from build123d import *

# Parameters (mm, degrees)
CROQUIS1_W              = 121.5
CROQUIS1_H              = 101
SALIENTE_EXTRUIR2_DEPTH = 4
SALIENTE_EXTRUIR3_DEPTH = 75
CROQUIS3_W              = 50
CROQUIS3_H              = 4
SALIENTE_EXTRUIR4_DEPTH = 75
CORTAR_EXTRUIR1_REACH   = 161.266
CROQUIS4_R              = 3.5
CROQUIS5_R              = 3.5
CORTAR_EXTRUIR2_DEPTH   = 4
CORTAR_EXTRUIR3_START   = -54.5
CORTAR_EXTRUIR3_DEPTH   = 109


with BuildPart() as part:
    # Croquis1 → Saliente-Extruir2 (new body)
    with BuildSketch(Plane(origin=(0, 0, 0), x_dir=(1, 0, 0), z_dir=(0, 1, 0))):
        Rectangle(CROQUIS1_W, CROQUIS1_H)
    extrude(amount=SALIENTE_EXTRUIR2_DEPTH)

    # Croquis2 → Saliente-Extruir3 (add)
    with BuildSketch(Plane(origin=(0, 0, 0), x_dir=(1, 0, 0), z_dir=(0, 1, 0))):
        Polygon((60.75, -50.5), (64.75, -50.5), (64.75, 54.5), (60.75, 54.5), (-64.75, 54.5), (-64.75, -50.5), (-60.75, -50.5), (-60.75, 50.5), (60.75, 50.5), align=None)
    extrude(amount=SALIENTE_EXTRUIR3_DEPTH)

    # Croquis3 → Saliente-Extruir4 (add)
    with BuildSketch(Plane(origin=(0, 0, 0), x_dir=(1, 0, 0), z_dir=(0, 1, 0))):
        with Locations((39.75, -52.5)):
            Rectangle(CROQUIS3_W, CROQUIS3_H)
    extrude(amount=SALIENTE_EXTRUIR4_DEPTH)

    # Cortar-Extruir1: up to this face of the body (flat: up to its plane)
    cortar_extruir1_end = Plane(part.part.faces().sort_by_distance((-64.75, 37.5, -2))[0])
    # Croquis4 → Cortar-Extruir1 (cut, up to the picked face)
    with BuildSketch(Plane(origin=(64.75, 0, 0), x_dir=(0, 0, -1), z_dir=(1, 0, 0)), mode=Mode.PRIVATE) as cortar_extruir1_sk1:
        with Locations((-35, 69.5)):
            Circle(CROQUIS4_R)
    cortar_extruir1_tool1 = split(extrude(cortar_extruir1_sk1.sketch, amount=-CORTAR_EXTRUIR1_REACH, mode=Mode.PRIVATE), bisect_by=cortar_extruir1_end, keep=Keep.BOTH, mode=Mode.PRIVATE)
    # Croquis4 → Cortar-Extruir1 (cut, up to the picked face)
    with BuildSketch(Plane(origin=(64.75, 0, 0), x_dir=(0, 0, -1), z_dir=(1, 0, 0)), mode=Mode.PRIVATE) as cortar_extruir1_sk2:
        with Locations((35, 9.5)):
            Circle(CROQUIS4_R)
    cortar_extruir1_tool2 = split(extrude(cortar_extruir1_sk2.sketch, amount=-CORTAR_EXTRUIR1_REACH, mode=Mode.PRIVATE), bisect_by=cortar_extruir1_end, keep=Keep.BOTH, mode=Mode.PRIVATE)
    # Croquis4 → Cortar-Extruir1 (cut, up to the picked face)
    with BuildSketch(Plane(origin=(64.75, 0, 0), x_dir=(0, 0, -1), z_dir=(1, 0, 0)), mode=Mode.PRIVATE) as cortar_extruir1_sk3:
        with Locations((-35, 9.5)):
            Circle(CROQUIS4_R)
    cortar_extruir1_tool3 = split(extrude(cortar_extruir1_sk3.sketch, amount=-CORTAR_EXTRUIR1_REACH, mode=Mode.PRIVATE), bisect_by=cortar_extruir1_end, keep=Keep.BOTH, mode=Mode.PRIVATE)
    # Croquis4 → Cortar-Extruir1 (cut, up to the picked face)
    with BuildSketch(Plane(origin=(64.75, 0, 0), x_dir=(0, 0, -1), z_dir=(1, 0, 0)), mode=Mode.PRIVATE) as cortar_extruir1_sk4:
        with Locations((35, 69.5)):
            Circle(CROQUIS4_R)
    cortar_extruir1_tool4 = split(extrude(cortar_extruir1_sk4.sketch, amount=-CORTAR_EXTRUIR1_REACH, mode=Mode.PRIVATE), bisect_by=cortar_extruir1_end, keep=Keep.BOTH, mode=Mode.PRIVATE)
    add(cortar_extruir1_tool1.solids().sort_by(Axis((64.75, 69.5, 35), (-1, 0, 0)))[0], mode=Mode.SUBTRACT)
    add(cortar_extruir1_tool2.solids().sort_by(Axis((64.75, 9.5, -35), (-1, 0, 0)))[0], mode=Mode.SUBTRACT)
    add(cortar_extruir1_tool3.solids().sort_by(Axis((64.75, 9.5, 35), (-1, 0, 0)))[0], mode=Mode.SUBTRACT)
    add(cortar_extruir1_tool4.solids().sort_by(Axis((64.75, 69.5, -35), (-1, 0, 0)))[0], mode=Mode.SUBTRACT)

    # Croquis5 → Cortar-Extruir2 (cut)
    with BuildSketch(Plane(origin=(0, 0, -54.5), x_dir=(-1, 0, 0), z_dir=(0, 0, -1))):
        with Locations((44.25, 69.5)):
            Circle(CROQUIS5_R)
        with Locations((44.25, 9.5)):
            Circle(CROQUIS5_R)
    extrude(amount=-CORTAR_EXTRUIR2_DEPTH, mode=Mode.SUBTRACT)

    # Croquis6 → Cortar-Extruir3 (cut)
    with BuildSketch(Plane.XY.offset(CORTAR_EXTRUIR3_START)):
        with BuildLine():
            Line((42.75, 69), (42.75, 75))
            Line((42.75, 75), (45.75, 75))
            Line((45.75, 75), (48.75, 75))
            Line((48.75, 75), (48.75, 69))
            ThreePointArc((48.75, 69), (45.75, 66), (42.75, 69))
        make_face()
        with BuildLine():
            ThreePointArc((48.75, 10), (47.871320344, 12.121320344), (45.75, 13))
            Line((45.75, 13), (45.75, 7))
            ThreePointArc((45.75, 7), (47.871320344, 7.878679656), (48.75, 10))
        make_face()
        with BuildLine():
            Line((45.75, 7), (45.75, 13))
            ThreePointArc((45.75, 13), (42.75, 10), (45.75, 7))
        make_face()
    extrude(amount=CORTAR_EXTRUIR3_DEPTH, mode=Mode.SUBTRACT)


solid = part.part
Design review of the part built by this model. Coordinates are the model's own, in mm. A direction names the side the tool comes from. Round coordinates to 2 decimals unless told otherwise and drop trailing zeros. Loops run counter-clockwise (first coordinate to the right, second up) from the corner with the lowest first, then second, coordinate; pieces in that order, holes last. Notation, with made-up numbers: M 82.25,50 L 105.25,50 A8 cw 105.25,54 Z; hole C 50.5,11.25 d10. An arc over 180 degrees is marked long. Answer as a JSON object with one key per item and string values.
Item 1: Machinability: for faces 4 (the flat face through (-37, 1, 50.5)), 5 (the flat face through (37, 39, 50.5)), 6 (the flat face through (39, 37, 54.5)), 7 (the flat face through (42.75, 72, -53)), 8 (the cylindrical face through (62.778, 69.654, 38.497)), which of the approach directions +Z, -Z, +X, -X, +Y, -Y give a long, thin tool a straight path to every point of the face, cutting with its end or side? Answer none if there is none.
Answer sheet:
{"face 4": "+Z, -X, +Y, -Y", "face 5": "+Y", "face 6": "+Z, +X, -X, +Y, -Y", "face 7": "+Z, -Z, +Y", "face 8": "+X, -X"}
Item 2: We need section D-D on z = -21. Give the boundary of the cut face in (x, y), and give its area (3 significant figures).
Answer sheet:
{"outline": "M -64.75,0 L 64.75,0 L 64.75,75 L 60.75,75 L 60.75,4 L -60.75,4 L -60.75,75 L -64.75,75 Z", "area": "1,090 mm^2"}
Item 3: We need section C-C on y = 23. Give the boundary of the cut face in (x, z).
Answer sheet:
{"outline": "M -64.75,-54.5 L 64.75,-54.5 L 64.75,54.5 L 14.75,54.5 L 14.75,50.5 L 60.75,50.5 L 60.75,-50.5 L -60.75,-50.5 L -60.75,50.5 L -64.75,50.5 Z"}
Item 4: Wall thickness on L1, parallel to Y at x = 62.7, z = -35; L2, parallel to Z at x = -61, y = 69; L3, parallel to Z at x = 63, y = 9: over which ranges is each line inside the solid? List them lowest first. Write a range as from..to.
Answer sheet:
{"L1": "y = 0..6, 13..66, 73..75", "L2": "z = -54.5..-38.46, -31.54..31.54, 38.46..50.5", "L3": "z = -54.5..-38.46, -31.54..31.54, 38.46..54.5"}
Item 5: Clearance check with flat-ended pins moving along their axes: P1, Ø6, axis at x = -14, y = 23, coming from the +Z side; P2, Ø6.5, axis at x = -44.25, y = 9.5, coming from the -Z side; P3, Ø3, axis at x = 45, z = 18, coming from the +Y side. State where each tip first meets the part, or that it passes through.
Answer sheet:
{"P1": "stops at z = -50.5", "P2": "passes through", "P3": "stops at y = 4"}
Item 6: We need section B-B on x = -44.25. Give the boundary of the cut face in (y, z).
Answer sheet:
{"outline": "M 0,-54.5 L 6,-54.5 L 6,-50.5 L 4,-50.5 L 4,50.5 L 0,50.5 Z; M 13,-54.5 L 66,-54.5 L 66,-50.5 L 13,-50.5 Z; M 73,-54.5 L 75,-54.5 L 75,-50.5 L 73,-50.5 Z"}
Item 7: The part is to be moulded in two halves that separate along Y. For faces 1 (the cylindrical face through (62.778, 69.654, -31.503)), 2 (the cylindrical face through (45.8, 66, 52.5)), 3 (the flat face through (14.75, 37, 53)), say which applies: pulls with the +Y half, pulls with the -Y half, needs draft (parallel to the pull), parting line crosses it, or undercut.
Answer sheet:
{"face 1": "undercut", "face 2": "pulls with the +Y half", "face 3": "needs draft"}
Item 8: We need section A-A on z = -35. Give the boundary of the cut face in (x, y).
Answer sheet:
{"outline": "M -64.75,0 L 64.75,0 L 64.75,6 L 60.75,6 L 60.75,4 L -60.75,4 L -60.75,6 L -64.75,6 Z; M -64.75,13 L -60.75,13 L -60.75,66 L -64.75,66 Z; M -64.75,73 L -60.75,73 L -60.75,75 L -64.75,75 Z; M 60.75,13 L 64.75,13 L 64.75,66 L 60.75,66 Z; M 60.75,73 L 64.75,73 L 64.75,75 L 60.75,75 Z"}
